Source: CAD feature listing. Evaluate the final solid. Frame: model axes, mm. A direction names the side the tool comes from. Coordinates: 2 decimals unless noted, no trailing zeros. Write each loop counter-clockwise with the first axis right and the second up, starting at its lowest first coordinate (ties: lowest second). Pieces come first, ordered by that corner, then holes. Notation, with made-up numbers: M -21.75,-6 L -9.75,-6 A17 ccw -9.75,17 Z; hole C 61.25,51.5 d6. An arc over 180 degrees is marked long. One line per item, written item: value. Start each with the question number.
Item 1: Mould query, pull axis X, two halves, no side actions, for faces 5 (the flat face through (-6, 2, 24.638)), 6 (the cylindrical face through (2.362, 4.845, 7.602)), 7 (the cylindrical face through (4.3, -4.224, 20.775)). Classes: released by +X, released by -X, zero draft, split by the parting line, or undercut.
Item 2: Cut plane C-C, the plane x = -6.5. Output: boundary loops of the cut face in (y, z), then the cut area to 3 significant figures.
Item 3: Pin query (flat end, axial travel): P1, Ø1, axis at y = -1.5, z = 18, coming from the -X side. Return the tip coordinate at first contact, or that it passes through.
Item 4: Cut plane A-A, the plane z = 18.5. Output: boundary loops of the cut face in (x, y) (3 decimals), then the cut area to 3 significant figures.
Item 5: Set-up query: faces 1 (the cylindrical face through (-4.359, 4.164, 20.775)), 2 (the flat face through (-0.1, -3.4, 17.018)), 3 (the cylindrical face through (3.604, -1.716, 20.775)), 4 (the cylindrical face through (6.04, -0.71, 20.77)). Return all of +Z, -Z, +X, -X, +Y, -Y with unobstructed straight access to the full face (end or side cutting, diameter ignored); none if empty.
Item 6: Ray query, L1, parallel to Z at x = 0, y = 6.75; L2, parallel to Y at x = 0, z = 13; L3, parallel to Y at x = -1.5, z = 12.25. Return the intervals inside material, ascending. Write a range as from..to.
Item 7: Cut plane D-D, the plane x = 2. State how many separate pieces and enclosed holes the cut face has, then the cut area to 3 significant figures.
Item 8: Cut plane B-B, the plane z = 10. Output: boundary loops of the cut face in (x, y), then the cut area to 3 significant figures.
```python
from build123d import *

# Parameters (mm, degrees)
F0_R        = 8.001
F0_R_2      = 3.048
F1_DEPTH    = 17.018
F3_W        = 16.002
F3_H        = 16.002
F4_DEPTH    = 17.018
F5_R        = 2.4765
F6_DEPTH    = 25.4
F7_T1_DEPTH = 57.023
F2_R        = 3.048
F8_DEPTH    = 25.4
F10_DEPTH   = 7.62
F11_SIZE    = 1.905


# Not quite as in the source:
# - a fillet or chamfer that OpenCascade refuses, or shapes differently, is made with other operations: its cross-section is extruded or revolved along the edge and cut away or added


with BuildPart() as f1:
    # F0 (on Top) → F1 (new body)
    with BuildSketch(Plane.XY):
        Circle(F0_R)
        Circle(F0_R_2, mode=Mode.SUBTRACT)
    extrude(amount=F1_DEPTH)

    # F3 (on Top) → F4 (join)
    with BuildSketch(Plane.XY):
        Rectangle(F3_W, F3_H)
    extrude(amount=F4_DEPTH)

    # F5 (on face) → F6 (cut)
    with BuildSketch(Plane.XZ.offset(8.001)):
        with Locations((0, 6.858)):
            Circle(F5_R)
    extrude(amount=-F6_DEPTH, mode=Mode.SUBTRACT)

    # F7: fillet of radius 8.001 on 4 edges, made by hand

    # F7_s2 → F7_t1 (cut)
    with BuildSketch(Plane.XY.offset(-20.0025)):
        with BuildLine():
            ThreePointArc((8.001, 0), (5.6575613563, -5.6575613563), (0, -8.001))
            Line((0, -8.001), (8.001, -8.001))
            Line((8.001, -8.001), (8.001, 0))
        make_face()
        with BuildLine():
            ThreePointArc((8.001, 0), (5.6575613563, 5.6575613563), (0, 8.001))
            Line((0, 8.001), (8.001, 8.001))
            Line((8.001, 8.001), (8.001, 0))
        make_face()
        with BuildLine():
            ThreePointArc((-8.001, 0), (-5.6575613563, -5.6575613563), (0, -8.001))
            Line((0, -8.001), (-8.001, -8.001))
            Line((-8.001, -8.001), (-8.001, 0))
        make_face()
        with BuildLine():
            ThreePointArc((0, 8.001), (-5.6575613563, 5.6575613563), (-8.001, 0))
            Line((-8.001, 0), (-8.001, 8.001))
            Line((-8.001, 8.001), (0, 8.001))
        make_face()
    extrude(amount=F7_T1_DEPTH, mode=Mode.SUBTRACT)

    # F2 (on face) → F8 (cut)
    with BuildSketch(Plane.XY.offset(17.018)):
        Circle(F2_R)
    extrude(amount=-F8_DEPTH, mode=Mode.SUBTRACT)

    # F9 (on face) → F10 (join)
    with BuildSketch(Plane.XY.offset(17.018)):
        with BuildLine():
            ThreePointArc((-3.0492599206, 2.589597302), (-4.3737921452, 4.1887242953), (-5.1697063492, 6.1065650953))
            ThreePointArc((-5.1697063492, 6.1065650953), (-7.2587471887, 3.3655), (-8.001, 0))
            ThreePointArc((-8.001, 0), (-6.0229894511, 0.6317175182), (-3.9466720244, 0.6540490669))
            ThreePointArc((-3.9466720244, 0.6540490669), (-3.6217185151, 1.6792007416), (-3.0492599206, 2.589597302))
        make_face()
        with BuildLine():
            ThreePointArc((3.0127388708, -2.6319963424), (4.3147732675, -4.2494941582), (5.0837832604, -6.1782804049))
            ThreePointArc((5.0837832604, -6.1782804049), (7.2109611489, -3.4667045316), (8.0002172314, -0.1119162637))
            ThreePointArc((8.0002172314, -0.1119162637), (6.0135638704, -0.7159039933), (3.9371372089, -0.7091902765))
            ThreePointArc((3.9371372089, -0.7091902765), (3.5978758903, -1.729696277), (3.0127388708, -2.6319963424))
        make_face()
    extrude(amount=F10_DEPTH)

    # F11
    f11_edges = [f1.edges().sort_by_distance(p)[0] for p in [
        (-3.048, 0, 0),
    ]]
    chamfer(f11_edges, length=F11_SIZE)


solid = f1.part
```
From the geometry:
1. face 5: zero draft
1. face 6: undercut
1. face 7: released by -X
2. outline: M -4.67,0 L 4.67,0 L 4.67,24.64 L 0.54,24.64 L 0.54,17.02 L -4.67,17.02 Z
2. area: 190 mm²
3. P1: stops at x = 3.46
4. outline: M -8.001,0 A6.985 cw -3.947,0.654 A4.239 cw -3.049,2.59 A6.985 cw -5.17,6.107 A8.001 ccw Z; M 3.013,-2.632 A6.985 cw 5.084,-6.178 A8.001 ccw 8,-0.112 A6.985 cw 3.937,-0.709 A4.239 cw Z
4. area: 33.1 mm²
5. face 1: +Z, +X, +Y
5. face 2: +Z
5. face 3: +Z, -X, +Y
5. face 4: +Z, +Y
6. L1: z = 0..4.38, 9.33..17.02
6. L2: y = -8..-3.05, 3.05..8
6. L3: y = -7.86..-2.65, 2.65..7.86
7. separate pieces: 4
7. enclosed holes: 0
7. area: 149 mm²
8. outline: C 0,0 d16; hole C 0,0 d6.1
8. area: 172 mm²
